```python
from build123d import *

# Parameters (mm, degrees)
F0_W     = 304.8
F0_H     = 361.95
F0_W_2   = 76.2
F0_H_2   = 152.4
F0_H_3   = 19.05
F1_DEPTH = 25.4
F3_DEPTH = 304.801


with BuildPart() as f1:
    # F0 (on Front) → F1 (new body)
    with BuildSketch(Plane.XZ):
        with Locations((0, 27.289911)):
            Rectangle(F0_W, F0_H)
        with Locations((-95.25, -58.435089)):
            Rectangle(F0_W_2, F0_H_2, mode=Mode.SUBTRACT)
        with Locations((0, -58.435089)):
            Rectangle(F0_W_2, F0_H_2, mode=Mode.SUBTRACT)
        with Locations((95.25, -58.435089)):
            Rectangle(F0_W_2, F0_H_2, mode=Mode.SUBTRACT)
        with Locations((-95.25, 113.014911)):
            Rectangle(F0_W_2, F0_H_2, mode=Mode.SUBTRACT)
        with Locations((0, 113.014911)):
            Rectangle(F0_W_2, F0_H_2, mode=Mode.SUBTRACT)
        with Locations((95.25, 113.014911)):
            Rectangle(F0_W_2, F0_H_2, mode=Mode.SUBTRACT)
        with Locations((0, -163.210089)):
            Rectangle(F0_W, F0_H_3)
    extrude(amount=F1_DEPTH)

    # F2 (on face) → F3 (cut, through all)
    with BuildSketch(Plane.YZ.offset(152.4)):
        with BuildLine():
            Line((0, -154.19948), (0, -153.143139))
            ThreePointArc((0, -153.143139), (-0.52817, -153.671309), (0, -154.19948))
        make_face()
    extrude(amount=-F3_DEPTH, mode=Mode.SUBTRACT)


solid = f1.part
```
Read the model definition and answer for the solid it produces. Units are mm, in the model's axes. A direction names the side the tool comes from. Coordinates: 2 decimals unless noted, no trailing zeros. Write each loop counter-clockwise with the first axis right and the second up, starting at its lowest first coordinate (ties: lowest second). Pieces come first, ordered by that corner, then holes. Notation, with made-up numbers: (7.5, 59) - (40.5, 59) arc R31 cw to (40.5, 96) - close; hole circle Ø1 at (14.25, 8). An arc over 180 degrees is marked (long way). Answer as a JSON object with one key per item and string values. Group by question number.
1. The mould has two halves that part along Z. Classify faces 3 (the flat face through (-2, -13, 208.265)), 4 (the flat face through (-57.15, -13, 112)), 5 (the flat face through (44, 0, -12)): +Z half, -Z half, draft (parallel to the pull), parting line (faces both ways), or undercut.
2. A cutting plane is placed at C-C (y = -20). Determine the outline of the cut face in (x, z).
3. Which of the six approach directions +Z, -Z, +X, -X, +Y, -Y give full straight-line access (tool end or side, diameter ignored) to faces 1 (the flat face through (-36, -25.4, 20)), 2 (the flat face through (-1, -13, 36.815))?
4. Consider L1, parallel to X at y = -2.75, z = 174.5; L2, parallel to Z at x = 24, y = -9.5. Determine where each line is inside the solid, lowest interval first. Write a range as [from, to].
5. A cutting plane is placed at A-A (z = -22). Determine the outline of the cut face in (x, y), plus the area to 3 significant figures.
6. A cutting plane is placed at B-B (x = -1.5). Determine the outline of the cut face in (y, z).
Worked out:
{
 "1": {"face 3": "+Z half", "face 4": "undercut", "face 5": "draft"},
 "2": {"outline": "(-152.4, -172.74) - (152.4, -172.74) - (152.4, 208.26) - (-152.4, 208.26) - close; hole (-133.35, -134.64) - (-57.15, -134.64) - (-57.15, 17.76) - (-133.35, 17.76) - close; hole (-133.35, 36.81) - (-57.15, 36.81) - (-57.15, 189.21) - (-133.35, 189.21) - close; hole (-38.1, -134.64) - (38.1, -134.64) - (38.1, 17.76) - (-38.1, 17.76) - close; hole (-38.1, 36.81) - (38.1, 36.81) - (38.1, 189.21) - (-38.1, 189.21) - close; hole (57.15, -134.64) - (133.35, -134.64) - (133.35, 17.76) - (57.15, 17.76) - close; hole (57.15, 36.81) - (133.35, 36.81) - (133.35, 189.21) - (57.15, 189.21) - close"},
 "3": {"face 1": "+Z, -Z, +X, -X, -Y", "face 2": "+Y, -Y"},
 "4": {"L1": "x = [-152.4, -133.35], [-57.15, -38.1], [38.1, 57.15], [133.35, 152.4]", "L2": "z = [-172.74, -134.64], [17.76, 36.81], [189.21, 208.26]"},
 "5": {"outline": "(-152.4, -25.4) - (-133.35, -25.4) - (-133.35, 0) - (-152.4, 0) - close; (-57.15, -25.4) - (-38.1, -25.4) - (-38.1, 0) - (-57.15, 0) - close; (38.1, -25.4) - (57.15, -25.4) - (57.15, 0) - (38.1, 0) - close; (133.35, -25.4) - (152.4, -25.4) - (152.4, 0) - (133.35, 0) - close", "area": "1,940 mm²"},
 "6": {"outline": "(-25.4, -172.74) - (0, -172.74) - (0, -154.2) arc R0.53 cw to (0, -153.14) - (0, -134.64) - (-25.4, -134.64) - close; (-25.4, 17.76) - (0, 17.76) - (0, 36.81) - (-25.4, 36.81) - close; (-25.4, 189.21) - (0, 189.21) - (0, 208.26) - (-25.4, 208.26) - close"}
}
